Input: part model. Units: mm. Frame: model coordinates. Face numbers are marked on the shaded views. A direction names the side the tool comes from. Give positions to 0.01 mm unless a question says otherwise; leave off trailing zeros. Loops run counter-clockwise (first coordinate to the right, second up) from the corner with the lowest first, then second, coordinate; pieces in that order, holes last. Notation, with made-up numbers: (-17, 16) -> (8, 16) arc R26 cw to (8, 47) -> close; hole circle Ø9 at (57, 38.25). An arc over 180 degrees is marked (long way). Answer as a JSON object with one key per item and string values.
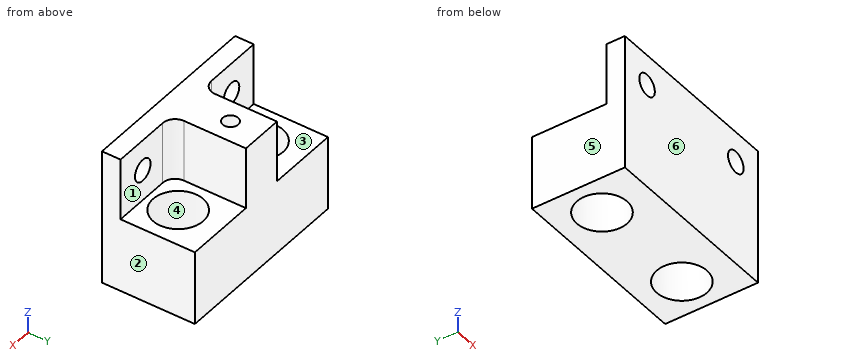
```python
from build123d import *

# Parameters (mm, degrees)
ESQUISSE1_W             = 30
ESQUISSE1_H             = 22
BOSS_EXTRU_1_DEPTH      = 15
ESQUISSE2_W             = 11.5
ESQUISSE2_H             = 10
ENL_V_MAT_EXTRU_2_DEPTH = 12
CONG_1_R                = 2
ESQUISSE3_R             = 4.05
ENL_V_MAT_EXTRU_3_DEPTH = 13
ENL_V_MAT_EXTRU_4_REACH = 5
ESQUISSE4_R             = 1.75
TROU_TARAUD_M31_D       = 2.5
TROU_TARAUD_M31_DEPTH   = 10
TROU_TARAUD_M31_TIP     = 0.751075774


with BuildPart() as part:
    # Esquisse1 → Boss.-Extru.1 (new body)
    with BuildSketch(Plane(origin=(0, 0, 0), x_dir=(1, 0, 0), z_dir=(0, 1, 0))):
        Rectangle(ESQUISSE1_W, ESQUISSE1_H)
    extrude(amount=BOSS_EXTRU_1_DEPTH)

    # Esquisse2 → Enlèv. mat.-Extru.2 (cut)
    with BuildSketch(Plane(origin=(0, 15, 0), x_dir=(1, 0, 0), z_dir=(0, 1, 0))):
        with Locations((-9.25, -6)):
            Rectangle(ESQUISSE2_W, ESQUISSE2_H)
        with Locations((9.25, -6)):
            Rectangle(ESQUISSE2_W, ESQUISSE2_H)
    extrude(amount=-ENL_V_MAT_EXTRU_2_DEPTH, mode=Mode.SUBTRACT)

    # Congé1
    cong_1_edges = [part.edges().sort_by_distance(p)[0] for p in [
        (-3.5, 3, 6),
        (3.5, 3, 6),
    ]]
    fillet(cong_1_edges, radius=CONG_1_R)

    # Esquisse3 → Enlèv. mat.-Extru.3 (cut, through all)
    with BuildSketch(Plane.XY.offset(1)):
        with Locations((-9, 8)):
            Circle(ESQUISSE3_R)
        with Locations((9, 8)):
            Circle(ESQUISSE3_R)
    extrude(amount=-ENL_V_MAT_EXTRU_3_DEPTH, mode=Mode.SUBTRACT)

    # Esquisse4 → Enlèv. mat.-Extru.4 (cut, up to next)
    with BuildSketch(Plane(origin=(0, 3, 0), x_dir=(1, 0, 0), z_dir=(0, 1, 0)), mode=Mode.PRIVATE) as enl_v_mat_extru_4_sk1:
        with Locations(Location((-10, -6, 0), (0, 0, 270))):  # turned: the seam where the file's is
            Circle(ESQUISSE4_R)
    enl_v_mat_extru_4_tool1 = extrude(enl_v_mat_extru_4_sk1.sketch, amount=-ENL_V_MAT_EXTRU_4_REACH, mode=Mode.PRIVATE) & part.part
    add(enl_v_mat_extru_4_tool1.solids().sort_by_distance((-10, 3, 6))[0], mode=Mode.SUBTRACT)
    # Esquisse4 → Enlèv. mat.-Extru.4 (cut, up to next)
    with BuildSketch(Plane(origin=(0, 3, 0), x_dir=(1, 0, 0), z_dir=(0, 1, 0)), mode=Mode.PRIVATE) as enl_v_mat_extru_4_sk2:
        with Locations(Location((10, -6, 0), (0, 0, 270))):  # turned: the seam where the file's is
            Circle(ESQUISSE4_R)
    enl_v_mat_extru_4_tool2 = extrude(enl_v_mat_extru_4_sk2.sketch, amount=-ENL_V_MAT_EXTRU_4_REACH, mode=Mode.PRIVATE) & part.part
    add(enl_v_mat_extru_4_tool2.solids().sort_by_distance((10, 3, 6))[0], mode=Mode.SUBTRACT)

    # Trou taraudé M31
    with Locations(Plane.XY.offset(11)):
        with Locations((0, 10)):
            Hole(TROU_TARAUD_M31_D / 2, depth=TROU_TARAUD_M31_DEPTH)
            with Locations((0, 0, -(TROU_TARAUD_M31_DEPTH + TROU_TARAUD_M31_TIP / 2))):  # 118° drill point
                Cone(0, TROU_TARAUD_M31_D / 2, TROU_TARAUD_M31_TIP, mode=Mode.SUBTRACT)


solid = part.part
```
Q1. Section C-C, the plane z = 9.75. Return the cut outline in (x, y), then the cut area to 3 significant figures.
Evaluation:
{"outline": "(-15, 0) -> (15, 0) -> (15, 3) -> (5.5, 3) arc R2 cw to (3.5, 5) -> (3.5, 15) -> (-3.5, 15) -> (-3.5, 5) arc R2 cw to (-5.5, 3) -> (-15, 3) -> close; hole circle Ø2.5 at (0, 10)", "area": "171 mm2"}
Q2. Ray query, line 1 along X through (y, z) = (0.9, 6); line 2 along X through (y, z) = (10, 6.5); line 3 along Y through (x, z) = (-9, -4). Return the intervals inside material, ascending.
Evaluation:
{"line 1": "x = -15 to -11.75, -8.25 to 8.25, 11.75 to 15", "line 2": "x = -3.5 to -1.25, 1.25 to 3.5", "line 3": "y = 0 to 3.95, 12.05 to 15"}
Q3. Pin query (flat end, axial travel): pin 1 (1.5 mm diameter, centred on x = -5.5, y = 7, fed in from +Z); pin 2 (10.5 mm diameter, centred on x = 11, z = 6.5, fed in from +Y); pin 3 (5 mm diameter, centred on y = 7.5, z = 6.5, fed in from -X); pin 4 (6.5 mm diameter, centred on x = 9, y = 8, fed in from -Z). Return the tip coordinate at first contact, or that it passes through.
Evaluation:
{"pin 1": "stops at z = 1", "pin 2": "stops at y = 3", "pin 3": "stops at x = -3.5", "pin 4": "passes through"}
Q4. Draft query along X for the marked faces 4, 5 and 6. Return one class per face: +X half, -X half, draft (parallel to the pull), parting line (faces both ways), or undercut.
Evaluation:
{"face 4": "undercut", "face 5": "-X half", "face 6": "draft"}
Q5. Section D-D, the plane x = -6.25. Return the cut outline in (y, z).
Evaluation:
{"outline": "(0, -11) -> (5.03, -11) -> (5.03, 1) -> (3, 1) -> (3, 11) -> (0, 11) -> close; (10.97, -11) -> (15, -11) -> (15, 1) -> (10.97, 1) -> close"}
Q6. Section B-B, the plane y = 13.5. Return the cut outline in (x, z).
Evaluation:
{"outline": "(-15, -11) -> (15, -11) -> (15, 1) -> (3.5, 1) -> (3.5, 11) -> (-3.5, 11) -> (-3.5, 1) -> (-15, 1) -> close"}
Q7. Section A-A, the plane y = 8. Return the cut outline in (x, z).
Evaluation:
{"outline": "(-15, -11) -> (-13.05, -11) -> (-13.05, 1) -> (-15, 1) -> close; (-4.95, -11) -> (4.95, -11) -> (4.95, 1) -> (3.5, 1) -> (3.5, 11) -> (-3.5, 11) -> (-3.5, 1) -> (-4.95, 1) -> close; (13.05, -11) -> (15, -11) -> (15, 1) -> (13.05, 1) -> close"}
Q8. Access query for the marked faces 1, 2 and 3. Directions: +Z, -Z, +X, -X, +Y, -Y. A direction counts if a zero-diameter tool reaches every point of the face in a straight line with its end or side. Return the directions, or none.
Evaluation:
{"face 1": "+Z, +X, +Y", "face 2": "+Z, -Z, +X, +Y, -Y", "face 3": "+Z, -X, +Y"}
